```python
from build123d import *

# Parameters (mm, degrees)
SKETCH1_R           = 2.25
BOSS_EXTRUDE1_DEPTH = 2.6
BOSS_EXTRUDE3_START = -3
SKETCH3_R           = 3.75
BOSS_EXTRUDE3_DEPTH = 3
CHAMFER2_SIZE       = 0.3
CHAMFER3_SIZE       = 0.5
SKETCH4_R           = 2.25
BOSS_EXTRUDE4_DEPTH = 12.5


with BuildPart() as part:
    # Sketch1 → Boss-Extrude1 (new body)
    with BuildSketch(Plane(origin=(0, 0, 0), x_dir=(0, 0, -1), z_dir=(1, 0, 0))):
        with BuildLine():
            Line((-21, -10), (6, -10))
            ThreePointArc((6, -10), (8.828427125, -8.828427125), (10, -6))
            Line((10, -6), (10, 19))
            ThreePointArc((10, 19), (8.828427125, 21.828427125), (6, 23))
            Line((6, 23), (-9.695652174, 23))
            ThreePointArc((-9.695652174, 23), (-11.354136506, 22.63997661), (-12.714074263, 21.62471486))
            Line((-12.714074263, 21.62471486), (-24.018422089, 8.62471486))
            ThreePointArc((-24.018422089, 8.62471486), (-24.746577662, 7.401126626), (-25, 6))
            Line((-25, 6), (-25, -6))
            ThreePointArc((-25, -6), (-23.828427125, -8.828427125), (-21, -10))
        make_face()
        with Locations((-15, 0)):
            Circle(SKETCH1_R, mode=Mode.SUBTRACT)
        with Locations((0, 17.25)):
            Circle(SKETCH1_R, mode=Mode.SUBTRACT)
        Circle(SKETCH1_R, mode=Mode.SUBTRACT)
    extrude(amount=BOSS_EXTRUDE1_DEPTH)

    # Sketch3 → Boss-Extrude3 (add)
    with BuildSketch(Plane(origin=(0, 0, 0), x_dir=(0, 0, -1), z_dir=(1, 0, 0)).offset(BOSS_EXTRUDE3_START)):
        with BuildLine():
            Line((-21, -10), (6, -10))
            ThreePointArc((6, -10), (8.828427125, -8.828427125), (10, -6))
            Line((10, -6), (10, 19))
            ThreePointArc((10, 19), (8.828427125, 21.828427125), (6, 23))
            Line((6, 23), (-9.695652174, 23))
            ThreePointArc((-9.695652174, 23), (-11.354136506, 22.63997661), (-12.714074263, 21.62471486))
            Line((-12.714074263, 21.62471486), (-24.018422089, 8.62471486))
            ThreePointArc((-24.018422089, 8.62471486), (-24.746577662, 7.401126626), (-25, 6))
            Line((-25, 6), (-25, -6))
            ThreePointArc((-25, -6), (-23.828427125, -8.828427125), (-21, -10))
        make_face()
        with Locations((-15, 0)):
            Circle(SKETCH3_R, mode=Mode.SUBTRACT)
        Circle(SKETCH3_R, mode=Mode.SUBTRACT)
        with Locations((0, 17.25)):
            Circle(SKETCH3_R, mode=Mode.SUBTRACT)
    extrude(amount=BOSS_EXTRUDE3_DEPTH)

    # Chamfer2
    chamfer2_edges = [part.edges().sort_by_distance(p)[0] for p in [
        (0, 0, 17.25),
        (0, 17.25, 2.25),
        (0, 0, 2.25),
        (0, 0, 18.75),
        (0, 0, 3.75),
        (0, 17.25, 3.75),
    ]]
    chamfer(chamfer2_edges, length=CHAMFER2_SIZE)

    # Chamfer3
    chamfer3_edges = [part.edges().sort_by_distance(p)[0] for p in [
        (-3, -8.828427125, 23.828427125),
        (-3, 0, 25),
        (-3, 7.401126626, 24.746577662),
        (-3, 15.12471486, 18.366248176),
        (-3, 22.63997661, 11.354136506),
        (-3, 23, 1.847826087),
        (-3, 21.828427125, -8.828427125),
        (-3, 6.5, -10),
        (-3, -8.828427125, -8.828427125),
        (-3, -10, 7.5),
        (-3, 17.25, 3.75),
        (-3, 0, 3.75),
        (-3, 0, 18.75),
    ]]
    chamfer(chamfer3_edges, length=CHAMFER3_SIZE)

    # Sketch4 → Boss-Extrude4 (add)
    with BuildSketch(Plane(origin=(2.6, 0, 0), x_dir=(0, 0, -1), z_dir=(1, 0, 0))):
        with BuildLine():
            Line((-21, -10), (6, -10))
            ThreePointArc((6, -10), (8.828427125, -8.828427125), (10, -6))
            Line((10, -6), (10, 6))
            ThreePointArc((10, 6), (8.828427125, 8.828427125), (6, 10))
            Line((6, 10), (-21, 10))
            ThreePointArc((-21, 10), (-23.828427125, 8.828427125), (-25, 6))
            Line((-25, 6), (-25, -6))
            ThreePointArc((-25, -6), (-23.828427125, -8.828427125), (-21, -10))
        make_face()
        Circle(SKETCH4_R, mode=Mode.SUBTRACT)
        with Locations((-15, 0)):
            Circle(SKETCH4_R, mode=Mode.SUBTRACT)
    extrude(amount=BOSS_EXTRUDE4_DEPTH)


solid = part.part
```
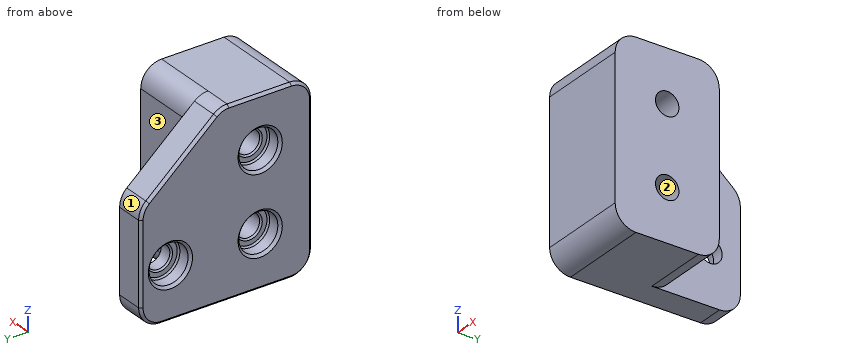
Geometry check sheet. Reference: the model listing, model coordinates, mm. Face numbers are marked on the shaded views. Coordinates: 2 decimals unless noted, no trailing zeros. Order: outer loops, then holes, each group sorted by start corner. A loop starts at its lowest first (then second) coordinate and runs counter-clockwise, first axis right, second up.
Q1. Draft check along Z on the marked faces 1, 2 and 3. Enter one of: released by +Z, released by -Z, zero draft, split by the parting line, or undercut.
Reply:
face 1: released by +Z
face 2: undercut
face 3: zero draft
Q2. Depth check by flat-ended pin: pin 1 Ø2 at (x, z) = (10.5, 20.5) entering from +Y; pin 2 Ø5.5 at (y, z) = (16.5, 0) entering from -X; pin 3 Ø3.5 at (y, z) = (-1.5, -1.5) entering from -X. Enter the tip coordinate at first touch or a pass-through.
Reply:
pin 1: stops at y = 10
pin 2: stops at x = -0.05
pin 3: stops at x = -2.62
Q3. Sectioned sample at C-C on y = 0. Give the number of separate pieces and of enclosed holes in the cut face, and give its area (3 significant figures).
Reply:
separate pieces: 3
enclosed holes: 0
area: 452 mm2
Q4. Sectioned sample at D-D on z = 7. Record the cut outline in (x, y), and give its area (3 significant figures).
Reply:
outline: (-3, -9.5) - (-2.5, -10) - (15.1, -10) - (15.1, 10) - (2.6, 10) - (2.6, 23) - (-2.5, 23) - (-3, 22.5) - close
area: 435 mm2
Q5. Sectioned sample at B-B on y = 17.25. Record the cut outline in (x, z).
Reply:
outline: (-3, -9.5) - (-2.5, -10) - (2.6, -10) - (2.6, -2.25) - (0.3, -2.25) - (0, -2.55) - (0, -3.45) - (-0.3, -3.75) - (-2.5, -3.75) - (-3, -4.25) - close; (-3, 4.25) - (-2.5, 3.75) - (-0.3, 3.75) - (0, 3.45) - (0, 2.55) - (0.3, 2.25) - (2.6, 2.25) - (2.6, 16.52) - (-2.5, 16.52) - (-3, 15.86) - close
Q6. Thickness scan on probe 1 along Y at (x, z) = (1.7, 0); probe 2 along Y at (x, z) = (-1.5, 0); probe 3 along Z at (x, y) = (12.25, -1). Record the ranges inside material, lowest first.
Reply:
probe 1: y = -10 to -2.25, 2.25 to 15, 19.5 to 23
probe 2: y = -10 to -3.75, 3.75 to 13.5, 21 to 23
probe 3: z = -10 to -2.02, 2.02 to 12.98, 17.02 to 25
Q7. Sectioned sample at A-A on x = 4.25. Record the cut outline in (y, z), and give its area (3 significant figures).
Reply:
outline: (-10, -6) arc R4 ccw to (-6, -10) - (6, -10) arc R4 ccw to (10, -6) - (10, 21) arc R4 ccw to (6, 25) - (-6, 25) arc R4 ccw to (-10, 21) - close; hole circle Ø4.5 at (0, 0); hole circle Ø4.5 at (0, 15)
area: 654 mm2
